```python
from build123d import *

# Parameters (mm, degrees)
F1_DEPTH = 2
F3_DEPTH = 3
F5_DEPTH = 2


with BuildPart() as f1:
    # F0 (on Front) → F1 (new body)
    with BuildSketch(Plane.XZ):
        with BuildLine():
            Line((-25, 0), (-2, 0))
            ThreePointArc((-2, 0), (-0.585786, 0.585786), (0, 2))
            Line((0, 2), (0, 19.5))
            ThreePointArc((0, 19.5), (-0.585786, 20.914214), (-2, 21.5))
            Line((-2, 21.5), (-25, 21.5))
            ThreePointArc((-25, 21.5), (-26.414214, 20.914214), (-27, 19.5))
            Line((-27, 19.5), (-27, 2))
            ThreePointArc((-27, 2), (-26.414214, 0.585786), (-25, 0))
        make_face()
    extrude(amount=F1_DEPTH)

    # F2 (on face) → F3 (join)
    with BuildSketch(Plane.XZ.offset(2)):
        with BuildLine():
            Line((-25, 0), (-17, 0))
            Line((-17, 0), (-17, 21.5))
            Line((-17, 21.5), (-25, 21.5))
            ThreePointArc((-25, 21.5), (-26.414214, 20.914214), (-27, 19.5))
            Line((-27, 19.5), (-27, 2))
            ThreePointArc((-27, 2), (-26.414214, 0.585786), (-25, 0))
        make_face()
        with BuildLine():
            Line((-10, 0), (-2, 0))
            ThreePointArc((-2, 0), (-0.585786, 0.585786), (0, 2))
            Line((0, 2), (0, 19.5))
            ThreePointArc((0, 19.5), (-0.585786, 20.914214), (-2, 21.5))
            Line((-2, 21.5), (-10, 21.5))
            Line((-10, 21.5), (-10, 0))
        make_face()
    extrude(amount=F3_DEPTH)

    # F4 (on face) → F5 (join)
    with BuildSketch(Plane.XZ.offset(5)):
        with BuildLine():
            Line((-17, 21.5), (-25, 21.5))
            ThreePointArc((-25, 21.5), (-26.414214, 20.914214), (-27, 19.5))
            Line((-27, 19.5), (-27, 2))
            ThreePointArc((-27, 2), (-26.414214, 0.585786), (-25, 0))
            Line((-25, 0), (-17, 0))
            Line((-17, 0), (-17, 21.5))
        make_face()
        with BuildLine():
            Line((-2, 21.5), (-17, 21.5))
            Line((-17, 21.5), (-17, 0))
            Line((-17, 0), (-2, 0))
            ThreePointArc((-2, 0), (-0.585786, 0.585786), (0, 2))
            Line((0, 2), (0, 19.5))
            ThreePointArc((0, 19.5), (-0.585786, 20.914214), (-2, 21.5))
        make_face()
    extrude(amount=F5_DEPTH)


solid = f1.part
```
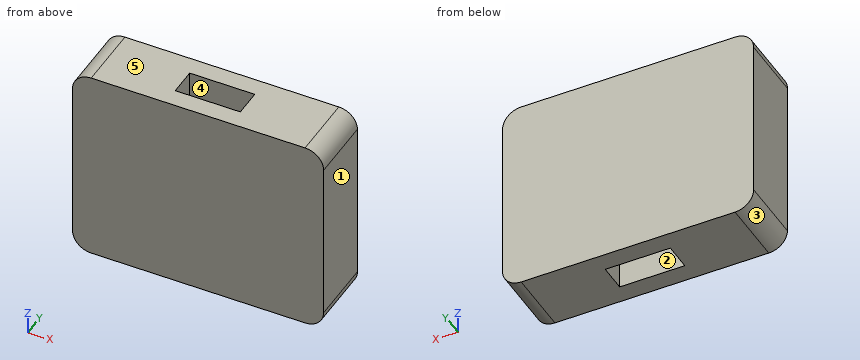
Could you check a few things on this model? Use its own coordinates, in mm. Face numbers are marked on the shaded views. A direction names the side the tool comes from. Round coordinates to 2 decimals unless told otherwise and drop trailing zeros. Loops run counter-clockwise (first coordinate to the right, second up) from the corner with the lowest first, then second, coordinate; pieces in that order, holes last. Notation, with made-up numbers: (4.25, 71.5) - (58.25, 71.5) arc R31 cw to (58.25, 107.5) - close; hole circle Ø11 at (27.5, 20.5). An arc over 180 degrees is marked (long way). Answer as CSV lines item,"result".
1. We'd pull the mould along X, two halves only. Please class the marked faces 1, 2 and 3: +X half, -X half, draft (parallel to the pull), parting line (faces both ways), or undercut.
Filled in:
face 1,"+X half"
face 2,"undercut"
face 3,"-X half"
2. I want a section at A-A on x = -10.75. List the corners of the cut face in (y, z) for me, then the cut area to 3 significant figures.
Filled in:
outline,"(-7, 0) - (-5, 0) - (-5, 21.5) - (-7, 21.5) - close; (-2, 0) - (0, 0) - (0, 21.5) - (-2, 21.5) - close"
area,"86.0 mm^2"
3. I want a section at B-B on y = -4. List the corners of the cut face in (x, z) for me.
Filled in:
outline,"(-27, 2) arc R2 ccw to (-25, 0) - (-17, 0) - (-17, 21.5) - (-25, 21.5) arc R2 ccw to (-27, 19.5) - close; (-10, 0) - (-2, 0) arc R2 ccw to (0, 2) - (0, 19.5) arc R2 ccw to (-2, 21.5) - (-10, 21.5) - close"
4. I want a section at C-C on z = 19. List the corners of the cut face in (x, y) for me, then the cut area to 3 significant figures.
Filled in:
outline,"(-27, -7) - (0, -7) - (0, 0) - (-27, 0) - close; hole (-17, -5) - (-10, -5) - (-10, -2) - (-17, -2) - close"
area,"168 mm^2"
5. Please list where these lines run through material, in increasing order: line 1 along X through (y, z) = (-3, 7.5); line 2 along Y through (x, z) = (-12.75, 19.75); line 3 along X through (y, z) = (-1, 19.75). Write a range as [from, to].
Filled in:
line 1,"x = [-27, -17], [-10, 0]"
line 2,"y = [-7, -5], [-2, 0]"
line 3,"x = [-26.98, -0.02]"
6. On a 3-axis mill with a long thin cutter (end or side, diameter ignored), from which of +Z, -Z, +X, -X, +Y, -Y can I reach the whole of each face in a straight line? I mean the marked faces 4 and 5. Say none if no direction works.
Filled in:
face 4,"+Z, -Z"
face 5,"+Z, +X, -X, +Y, -Y"
